from build123d import *

# Parameters (mm, degrees)
SKETCH_6_R      = 6
EXTRUDE_3_DEPTH = 3.9
SKETCH_7_R      = 5.8
EXTRUDE_4_DEPTH = 9.5
SKETCH_8_R      = 5.25
EXTRUDE_5_DEPTH = 13.7
SKETCH_9_W      = 4.89861288
SKETCH_9_H      = 0.5003769
SKETCH_9_H_2    = 0.495607413
EXTRUDE_6_DEPTH = 5


with BuildPart() as part:
    # Эскиз5 → Повернуть1 (revolve)
    with BuildSketch(Plane.XY, mode=Mode.PRIVATE) as revolve_1_sk:
        Polygon((-7.2, 7.5), (-9.1, 0), (0, 0), (0, 7.5), align=None)
    revolve(revolve_1_sk.sketch.rotate(Axis((0, 0, 0), (0, 1, 0)), 270), axis=Axis((0, 0, 0), (0, 1, 0)))

    # Эскиз6 → Бобышка-Вытянуть3 (add)
    with BuildSketch(Plane(origin=(0, 7.5, 0), x_dir=(1, 0, 0), z_dir=(0, 1, 0))):
        with Locations(Location((0, 0, 0), (0, 0, 90))):
            Circle(SKETCH_6_R)
    extrude(amount=EXTRUDE_3_DEPTH)

    # Эскиз7 → Бобышка-Вытянуть4 (add)
    with BuildSketch(Plane.XZ):
        with Locations(Location((0, 0, 0), (0, 0, 90))):
            Circle(SKETCH_7_R)
    extrude(amount=EXTRUDE_4_DEPTH)

    # Эскиз8 → Бобышка-Вытянуть5 (add)
    with BuildSketch(Plane.XZ.offset(9.5)):
        with Locations(Location((0, 0, 0), (0, 0, 90))):
            Circle(SKETCH_8_R)
    extrude(amount=EXTRUDE_5_DEPTH)

    # Эскиз9 → Бобышка-Вытянуть6 (add)
    with BuildSketch(Plane(origin=(0, -23.2, 0), x_dir=(-1, 0, 0), z_dir=(0, -1, 0))):
        with Locations((-0.000422971, 2.45018845)):
            Rectangle(SKETCH_9_W, SKETCH_9_H)
        with Locations((-0.000422971, -2.447803707)):
            Rectangle(SKETCH_9_W, SKETCH_9_H_2)
    extrude(amount=EXTRUDE_6_DEPTH)


solid = part.part
Design review of the part built by this model. Coordinates are the model's own, in mm. A direction names the side the tool comes from. Round coordinates to 2 decimals unless told otherwise and drop trailing zeros. Loops run counter-clockwise (first coordinate to the right, second up) from the corner with the lowest first, then second, coordinate; pieces in that order, holes last. Notation, with made-up numbers: (85.25, -20.75) - (143.25, -20.75) arc R18 ccw to (143.25, -8.75) - close; hole circle Ø10 at (44.25, -25.5). An arc over 180 degrees is marked (long way). One line per question, with ' | ' between items.
1. We need section C-C, the plane y = -15. State the section outline as (x, z) points, and give its area (3 significant figures).
Results are:
outline: circle Ø10.5 at (0, 0) | area: 86.6 mm²
2. For L1, parallel to Z at x = -1.5, y = -24; L2, parallel to X at y = -21.5, z = 0; L3, parallel to Z at x = 0.25, y = 9.5, list the stretches that pass through material, from the lowest coordinate up. Write a range as [from, to].
Results are:
L1: z = [-2.7, -2.2], [2.2, 2.7] | L2: x = [-5.25, 5.25] | L3: z = [-5.99, 5.99]
3. Draft analysis for pull direction Z (two halves, no side actions). For faces 1 (the face through (6, 0, 0)), 2 (the face through (0, -26, 2.696)), 3 (the face through (-1.802, 9.423, -5.723)), 4 (the face through (0, -26, -2.2)), state which applies: released by +Z, released by -Z, zero draft, split by the parting line, or undercut.
Results are:
face 1: zero draft | face 2: released by +Z | face 3: split by the parting line | face 4: undercut
4. We need section A-A, the plane z = 0. State the section outline as (x, y) points.
Results are:
outline: (-9.1, 0) - (-5.8, 0) - (-5.8, -9.5) - (-5.25, -9.5) - (-5.25, -23.2) - (5.25, -23.2) - (5.25, -9.5) - (5.8, -9.5) - (5.8, 0) - (9.1, 0) - (7.2, 7.5) - (6, 7.5) - (6, 11.4) - (-6, 11.4) - (-6, 7.5) - (-7.2, 7.5) - close
5. We need section B-B, the plane x = 0. State the section outline as (y, z) points.
Results are:
outline: (-28.2, -2.7) - (-23.2, -2.7) - (-23.2, -5.25) - (-9.5, -5.25) - (-9.5, -5.8) - (0, -5.8) - (0, -9.1) - (7.5, -7.2) - (7.5, -6) - (11.4, -6) - (11.4, 6) - (7.5, 6) - (7.5, 7.2) - (0, 9.1) - (0, 5.8) - (-9.5, 5.8) - (-9.5, 5.25) - (-23.2, 5.25) - (-23.2, 2.7) - (-28.2, 2.7) - (-28.2, 2.2) - (-23.2, 2.2) - (-23.2, -2.2) - (-28.2, -2.2) - close
6. Clearance check with flat-ended pins moving along their axes: P1, Ø1.5, axis at x = 0.5, y = -26, coming from the -Z side; P2, Ø1.5, axis at x = -5.5, z = 5, coming from the +Y side; P3, Ø1.5, axis at x = 1, y = -25, coming from the +Z side. State where each tip first meets the part, or that it passes through.
Results are:
P1: stops at z = -2.7 | P2: stops at y = 7.5 | P3: stops at z = 2.7
7. We need section D-D, the plane y = -1. State the section outline as (x, z) points, and give its area (3 significant figures).
Results are:
outline: circle Ø11.6 at (0, 0) | area: 106 mm²
8. For faces 5 (the face through (0, -26, 2.2)), 6 (the face through (-6, 7.5, -2)), 7 (the face through (-1.6, -16.3, 5)), list the 3-axis set-ups (+Z, -Z, +X, -X, +Y, -Y) from which the entire face can be reached by the end or side of a thin tool; tool diameter is ignored.
Results are:
face 5: +X, -X, -Y | face 6: +Y | face 7: -Y
